Study the drawing (mm; zero at the part's minimum x, y, z) and answer. Coordinates: 2 decimals unless noted, no trailing zeros. Order: outer loops, then holes, each group sorted by start corner. A loop starts at its lowest first (then second) coordinate and runs counter-clockwise, first axis right, second up.
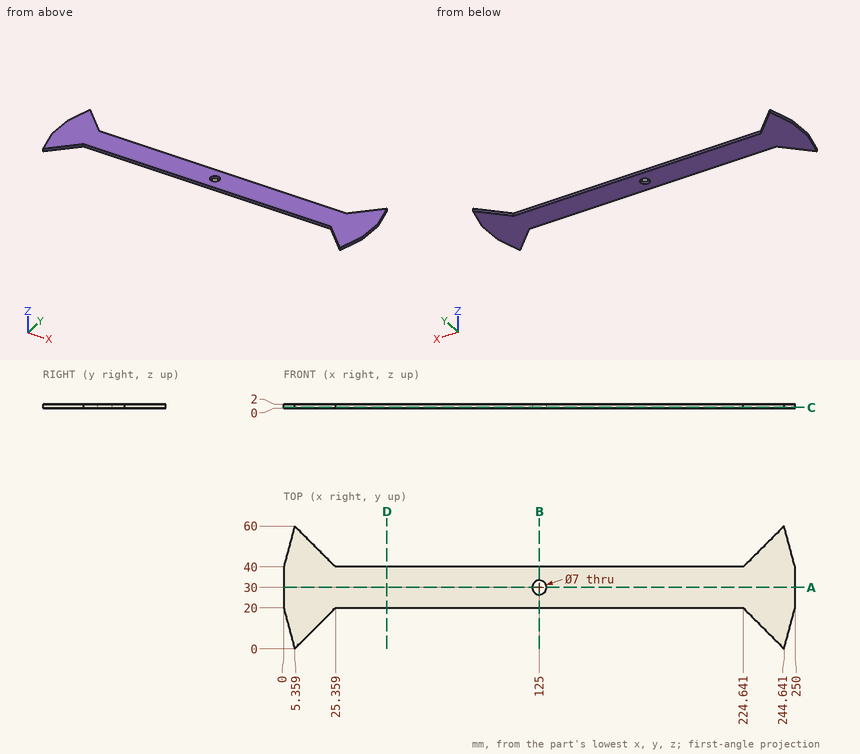
(1) Each of these flat-tipped pins is pushed along its axis until it touches: pin 1 Ø12 at (x, y) = (37, 51) entering from -Z; pin 2 Ø1 at (x, z) = (85, 0.5) entering from -Y; pin 3 Ø0.6 at (x, z) = (124, 1.5) entering from +Y. Where does it stop, or does it pass through?
(2) Find section A-A (y = 30). Write down the section's boundary in (x, z).
(3) Find section B-B (x = 125). Write down the section's boundary in (y, z), and give its area (3 significant figures).
(4) Consider line 1 (Y direction, x = 125, z = 1.6); line 2 (X direction, y = 54, z = 1.75); line 3 (X direction, y = 3, z = 1.15). Determine where each line is inside the solid, lowest interval first.
(5) Find section C-C (z = 0.3). Write down the section's boundary in (x, y), and give its area (3 significant figures).
(6) Find section D-D (x = 50.5). Write down the section's boundary in (y, z).
Findings below:
1. pin 1: passes through
1. pin 2: stops at y = 20
1. pin 3: stops at y = 40
2. outline: (0, 0) - (121.5, 0) - (121.5, 2) - (0, 2) - close; (128.5, 0) - (250, 0) - (250, 2) - (128.5, 2) - close
3. outline: (20, 0) - (26.5, 0) - (26.5, 2) - (20, 2) - close; (33.5, 0) - (40, 0) - (40, 2) - (33.5, 2) - close
3. area: 26.0 mm2
4. line 1: y = 20 to 26.5, 33.5 to 40
4. line 2: x = 3.75 to 11.36, 238.64 to 246.25
4. line 3: x = 4.56 to 8.36, 241.64 to 245.44
5. outline: (0, 20) - (5.36, 0) - (25.36, 20) - (224.64, 20) - (244.64, 0) - (250, 20) - (250, 40) - (244.64, 60) - (224.64, 40) - (25.36, 40) - (5.36, 60) - (0, 40) - close; hole circle Ø7 at (125, 30)
5. area: 5,980 mm2
6. outline: (20, 0) - (40, 0) - (40, 2) - (20, 2) - close
